Autodesk Inventor part; units mm, degrees
ref_plane "YZ Plane" through (0, 0, 0) normal (1, 0, 0) x (0, 1, 0)
ref_plane "XZ Plane" through (0, 0, 0) normal (0, 1, 0) x (-1, 0, 0)
ref_plane "XY Plane" through (0, 0, 0) normal (0, 0, 1) x (1, 0, 0)
sketch "スケッチ1" plane through (0, 0, 0) normal (1, 0, 0) x (0, 1, 0)
  line L0 (-5, -20) -> (5, -20)
  line L1 (5, -20) -> (5, 20)
  line L2 (5, 20) -> (-5, 20)
  line L3 (-5, 20) -> (-5, -20)
  line L4 (-5, -20) -> (5, 20) construction
  line L5 (5, -20) -> (-5, 20) construction
  point P0 (0, 0)
  dimension "d0" = 10
  dimension "d1" = 40
extrude "押し出し1" add sketch "スケッチ1" along normal blind 10
shell "シェル1" thickness 1 removed faces 4 at (3.3333, 1.6667, 20) at (3.3333, 5, -6.6667) at (3.3333, -1.6667, -20) at (10, -1.6667, 6.6667)
sketch "スケッチ2" plane through (0, 0, 0) normal (-1, 0, 0) x (0, 0, 1)
  line L0 (-20, -5) -> (-20, 5)
  line L1 (20, 5) -> (20, -4.2502)
  line L2 (-20, 5) -> (20, 5)
  point P0 (0, 0)
  point P1 (-15, 0)
  point P2 (15, 0)
  dimension "d5" = 5
  dimension "d6" = 5
  dimension "d14" = 5
hole "穴1" at (0, 0, -15) at (0, 0, 15) direction (1, 0, 0) diameter 3 end through all
sketch "スケッチ3" plane through (0, -5, -20) normal (0, -1, 0) x (1, 0, 0)
  line L0 (3, 4) -> (3, 36)
  arc A0 (7, 36) -> (3, 36) centre (5, 36) ccw
  line L1 (7, 36) -> (7, 4)
  arc A1 (3, 4) -> (7, 4) centre (5, 4) ccw
  line L2 (0, 0) -> (10, 0)
  line L3 (10, 40) -> (10, 0)
  line L4 (0, 40) -> (10, 40)
  point P0 (0, 20)
  dimension "d15" = 2
  dimension "d16" = 4
  dimension "d17" = 5
  dimension "d18" = 4
extrude "押し出し2" cut sketch "スケッチ3" against normal blind 1
properties part number "palmrest_L_small" material "アルミニウム 6061"
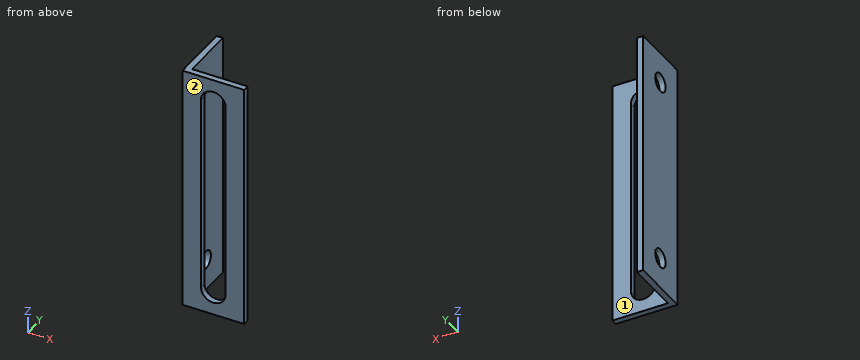
Input: part model. Units: mm. Frame: model coordinates. Face numbers are marked on the shaded views. A direction names the side the tool comes from. Coordinates: 2 decimals unless noted, no trailing zeros. Write each loop counter-clockwise with the first axis right and the second up, starting at its lowest first coordinate (ties: lowest second). Pieces come first, ordered by that corner, then holes.
1) Section A-A on y = 0. Output: boundary loops of the cut face in (x, z), and give its area (3 significant figures).
2) Pin query (flat end, axial travel): pin 1 Ø6 at (y, z) = (1.5, -14.5) entering from +X; pin 2 Ø5 at (y, z) = (-4, 6) entering from -X. Return the tip coordinate at first contact, or that it passes through.
3) Material intervals for line 1 along Z through (x, y) = (0.7, 0); line 2 along Y through (x, z) = (0.2, -15); line 3 along X through (y, z) = (-3, 6), sorted ascending.
4) Section C-C on x = 5. Output: boundary loops of the cut face in (y, z).
5) Section B-B on z = 5.5. Output: boundary loops of the cut face in (x, y), and give its area (3 significant figures).
6) Set-up query: the marked faces 1 and 2. Return all of +Z, -Z, +X, -X, +Y, -Y with unobstructed straight access to the full face (end or side cutting, diameter ignored); none if empty.
7) Section D-D on z = 15. Output: boundary loops of the cut face in (x, y).
Check result:
1. outline: (0, -20) - (1, -20) - (1, -16.5) - (0, -16.5) - close; (0, -13.5) - (1, -13.5) - (1, 13.5) - (0, 13.5) - close; (0, 16.5) - (1, 16.5) - (1, 20) - (0, 20) - close
1. area: 34.0 mm2
2. pin 1: stops at x = 1
2. pin 2: stops at x = 0
3. line 1: z = -20 to -16.5, -13.5 to 13.5, 16.5 to 20
3. line 2: y = -5 to -1.5, 1.5 to 5
3. line 3: x = 0 to 1
4. outline: (-5, -20) - (-4, -20) - (-4, -18) - (-5, -18) - close; (-5, 18) - (-4, 18) - (-4, 20) - (-5, 20) - close
5. outline: (0, -5) - (3, -5) - (3, -4) - (1, -4) - (1, 5) - (0, 5) - close; (7, -5) - (10, -5) - (10, -4) - (7, -4) - close
5. area: 15.0 mm2
6. face 1: +Z, -Z, +X, +Y
6. face 2: +Z, -Z, +X, -X, -Y
7. outline: (0, -5) - (3, -5) - (3, -4) - (1, -4) - (1, -1.5) - (0, -1.5) - close; (0, 1.5) - (1, 1.5) - (1, 5) - (0, 5) - close; (7, -5) - (10, -5) - (10, -4) - (7, -4) - close
